Here's how the part is built. I have some questions about the finished solid (model axes, mm). Face numbers are marked on the shaded views. A direction names the side the tool comes from. Round coordinates to 2 decimals unless told otherwise and drop trailing zeros. Order: outer loops, then holes, each group sorted by start corner. A loop starts at its lowest first (then second) coordinate and runs counter-clockwise, first axis right, second up.
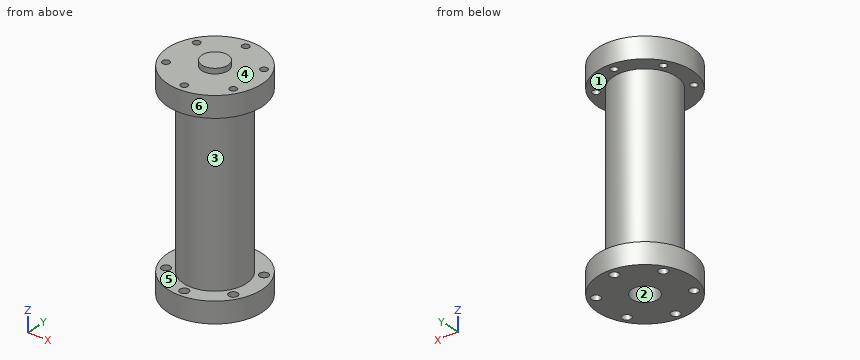
```python
from build123d import *

# Parameters (mm, degrees)
SKETCH1_R                      = 45
BOSS_EXTRUDE1_DEPTH            = 20
SKETCH2_R                      = 30
BOSS_EXTRUDE2_DEPTH            = 160
SKETCH3_R                      = 45
BOSS_EXTRUDE3_DEPTH            = 20
SKETCH4_R                      = 12.5
BOSS_EXTRUDE4_DEPTH            = 5
M8X1_25_TAPPED_HOLE1_REACH     = 202
M8X1_25_TAPPED_HOLE1_BORE_R    = 3.4
CIRPATTERN1_COUNT              = 6
F_8_5_8_5_DIAMETER_HOLE1_D     = 8.5
F_8_5_8_5_DIAMETER_HOLE1_DEPTH = 20.001
CIRPATTERN2_COUNT              = 6
SKETCH11_R                     = 12.5
CUT_EXTRUDE1_DEPTH             = 60


with BuildPart() as part:
    # Sketch1 → Boss-Extrude1 (new body)
    with BuildSketch(Plane.XY):
        Circle(SKETCH1_R)
    extrude(amount=BOSS_EXTRUDE1_DEPTH)

    # Sketch2 → Boss-Extrude2 (add)
    with BuildSketch(Plane(origin=(0, 0, 0), x_dir=(-1, 0, 0), z_dir=(0, 0, -1))):
        Circle(SKETCH2_R)
    extrude(amount=BOSS_EXTRUDE2_DEPTH)

    # Sketch3 → Boss-Extrude3 (add)
    with BuildSketch(Plane(origin=(0, 0, -160), x_dir=(-1, 0, 0), z_dir=(0, 0, -1))):
        with Locations(Location((0, 0, 0), (0, 0, 180))):  # turned: the seam where the file's is
            Circle(SKETCH3_R)
    extrude(amount=BOSS_EXTRUDE3_DEPTH)

    # Sketch4 → Boss-Extrude4 (add)
    with BuildSketch(Plane.XY.offset(20)):
        Circle(SKETCH4_R)
    extrude(amount=BOSS_EXTRUDE4_DEPTH)

    # M8x1.25 Tapped Hole1 bore → M8x1.25 Tapped Hole1 (cut, up to next)
    with BuildSketch(Plane.XY.offset(20), mode=Mode.PRIVATE) as m8x1_25_tapped_hole1_sk1:
        with Locations((0, 37.5)):
            Circle(M8X1_25_TAPPED_HOLE1_BORE_R)
    m8x1_25_tapped_hole1_tool1 = extrude(m8x1_25_tapped_hole1_sk1.sketch, amount=-M8X1_25_TAPPED_HOLE1_REACH, mode=Mode.PRIVATE) & part.part
    m8x1_25_tapped_hole1 = m8x1_25_tapped_hole1_tool1.solids().sort_by_distance((0, 37.5, 20))[0]
    add(m8x1_25_tapped_hole1, mode=Mode.SUBTRACT)

    # CirPattern1: M8x1.25 Tapped Hole1 ×6 about axis
    cirpattern1_axis = Axis((0, 0, 0), (0, 0, 1))
    for i in range(1, CIRPATTERN1_COUNT):
        add(m8x1_25_tapped_hole1.rotate(cirpattern1_axis, i * 360 / CIRPATTERN1_COUNT), mode=Mode.SUBTRACT)

    # Ø8.5 (8.5) Diameter Hole1
    with Locations(Plane(origin=(0, 0, -180), x_dir=(-1, 0, 0), z_dir=(0, 0, -1))):
        with Locations((0, 37.5)):
            f_8_5_8_5_diameter_hole1 = Hole(F_8_5_8_5_DIAMETER_HOLE1_D / 2, depth=F_8_5_8_5_DIAMETER_HOLE1_DEPTH)

    # CirPattern2: Ø8.5 (8.5) Diameter Hole1 ×6 about axis
    cirpattern2_axis = Axis((0, 0, 0), (0, 0, 1))
    for i in range(1, CIRPATTERN2_COUNT):
        add(f_8_5_8_5_diameter_hole1.rotate(cirpattern2_axis, i * 360 / CIRPATTERN2_COUNT), mode=Mode.SUBTRACT)

    # Sketch11 → Cut-Extrude1 (cut)
    with BuildSketch(Plane(origin=(0, 0, -180), x_dir=(-1, 0, 0), z_dir=(0, 0, -1))):
        with Locations(Location((0, 0, 0), (0, 0, 180))):  # turned: the seam where the file's is
            Circle(SKETCH11_R)
    extrude(amount=-CUT_EXTRUDE1_DEPTH, mode=Mode.SUBTRACT)


solid = part.part
```
1) I need wall thicknesses on line 1 (Z direction, x = 34, y = 14); line 2 (Z direction, x = 12, y = -14); line 3 (Z direction, x = 8, y = 0). Which ranges of each line are inside material? Lowest first, please.
2) If we section it at C-C (x = 0): Give the number of separate pieces and of enclosed holes in the cut face, plus the area to 3 significant figures.
3) I'm going to push flat-ended pins straight in: pin 1 (5 mm diameter, centred on x = -27, z = -124.5, fed in from +Y); pin 2 (10 mm diameter, centred on y = -17.5, z = -18, fed in from +X); pin 3 (6 mm diameter, centred on x = -6.5, z = -82.5, fed in from +Y). Where does each tip first touch, or does it pass through?
4) If we section it at D-D (y = 18.75): Write out the boundary of the cut face in (x, z).
5) If we section it at A-A (y = 0): Write out the boundary of the cut face in (x, z).
6) For the marked faces 4, 5 and 6, which set-ups out of +Z, -Z, +X, -X, +Y, -Y let a thin tool reach every point of the face, with its end or its side?
7) We'd pull the mould along Y, two halves only. Please class the marked faces 1, 2 and 3: +Y half, -Y half, draft (parallel to the pull), parting line (faces both ways), or undercut.
8) If we section it at B-B (y = 37.5): Write out the boundary of the cut face in (x, z).
Solutions:
1. line 1: z = -180 to -160, 0 to 20
1. line 2: z = -180 to 20
1. line 3: z = -120 to 25
2. separate pieces: 5
2. enclosed holes: 0
2. area: 11,200 mm2
3. pin 1: stops at y = 17.31
3. pin 2: stops at x = 27.27
3. pin 3: stops at y = 29.8
4. outline: (-40.91, -180) - (-36.73, -180) - (-36.73, -160) - (-40.91, -160) - close; (-40.91, 0) - (-35.88, 0) - (-35.88, 20) - (-40.91, 20) - close; (-29.08, 0) - (-23.42, 0) - (-23.42, -160) - (-28.23, -160) - (-28.23, -180) - (28.23, -180) - (28.23, -160) - (23.42, -160) - (23.42, 0) - (29.08, 0) - (29.08, 20) - (-29.08, 20) - close; (35.88, 0) - (40.91, 0) - (40.91, 20) - (35.88, 20) - close; (36.73, -180) - (40.91, -180) - (40.91, -160) - (36.73, -160) - close
5. outline: (-45, -180) - (-12.5, -180) - (-12.5, -120) - (12.5, -120) - (12.5, -180) - (45, -180) - (45, -160) - (30, -160) - (30, 0) - (45, 0) - (45, 20) - (12.5, 20) - (12.5, 25) - (-12.5, 25) - (-12.5, 20) - (-45, 20) - (-45, 0) - (-30, 0) - (-30, -160) - (-45, -160) - close
6. face 4: +Z
6. face 5: none
6. face 6: +Z, -Z
7. face 1: draft
7. face 2: undercut
7. face 3: parting line
8. outline: (-24.87, -180) - (-4.25, -180) - (-4.25, -160) - (-24.87, -160) - close; (-24.87, 0) - (-3.4, 0) - (-3.4, 20) - (-24.87, 20) - close; (3.4, 0) - (24.87, 0) - (24.87, 20) - (3.4, 20) - close; (4.25, -180) - (24.87, -180) - (24.87, -160) - (4.25, -160) - close
